Geometry check sheet. Reference: drawing and pictorial views, mm from the part's lowest x, y, z. A direction names the side the tool comes from. Coordinates: 2 decimals unless noted, no trailing zeros. Loops run counter-clockwise (first coordinate to the right, second up) from the corner with the lowest first, then second, coordinate; pieces in that order, holes last. Notation, with made-up numbers: M -36.5,40 L -22.5,40 A31 ccw -22.5,70 Z; hole C 56.5,81 d5. An arc over 180 degrees is marked long. Write item = value, one per line. Start each with the question number.
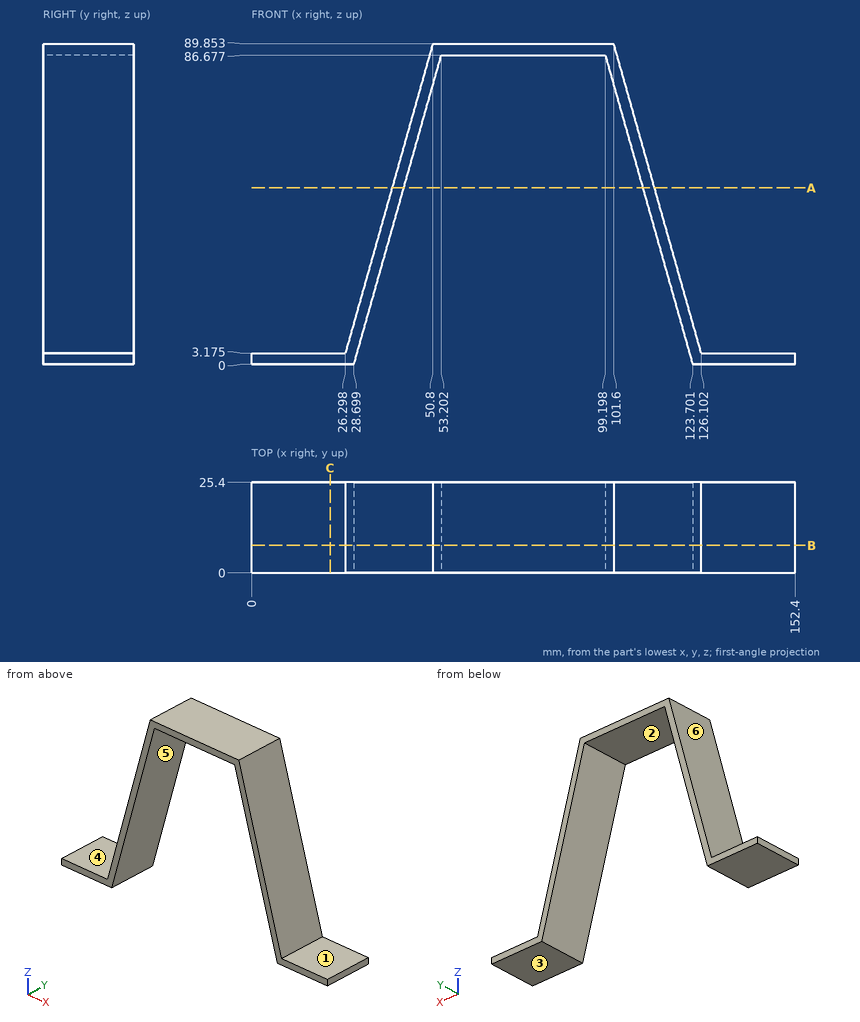
Q1. Scan lines: L1, parallel to Z at x = 13, y = 4.75 (1 decimal); L2, parallel to X at y = 8.5, z = 61 (1 decimal); L3, parallel to X at y = 1.75, z = 20 (1 decimal). Record each from-to range of solid material in increasing order. Write a range as [from, to].
Q2. Mould release check, pull along X, two halves, no side actions. Record for the marked faces 4, 5 and 6: +X half, -X half, draft (parallel to the pull), parting line (faces both ways), or undercut.
Q3. Sectioned sample at C-C on x = 22. Record the cut outline in (y, z) (1 decimal).
Q4. Gauge pin test, flat ends, axial feed: pin 1 (7.5 mm diameter, centred on x = 87.5, y = 16, fed in from -Z); pin 2 (1.5 mm diameter, centred on y = 17.5, z = 55.5, fed in from -X); pin 3 (12 mm diameter, centred on y = 9, z = 41, fed in from -X); pin 4 (12 mm diameter, centred on x = 96, z = 75, fed in from -Y). Record the tip position at first contact, or that the pin passes through.
Q5. Sectioned sample at B-B on y = 7.75. Record the cut outline in (x, z) (1 decimal).
Q6. Set-up check for the marked faces 1, 2 and 3: record each of +Z, -Z, +X, -X, +Y, -Y from which the full face is reachable in a straight line by a thin tool's end or side.
Q7. Sectioned sample at A-A on z = 49.5. Record the cut outline in (x, y).
Solutions:
q1.L1 = [0, 3.2]
q1.L2 = [42.6, 45.9], [106.5, 109.8]
q1.L3 = [31.1, 34.4], [118, 121.3]
q2.face_4 = draft
q2.face_5 = undercut
q2.face_6 = -X half
q3.outline = M 0,0 L 25.4,0 L 25.4,3.2 L 0,3.2 Z
q4.pin_1 = 86.68
q4.pin_2 = 40.88
q4.pin_3 = 35.29
q4.pin_4 = through
q5.outline = M 0,0 L 28.7,0 L 53.2,86.7 L 99.2,86.7 L 123.7,0 L 152.4,0 L 152.4,3.2 L 126.1,3.2 L 101.6,89.9 L 50.8,89.9 L 26.3,3.2 L 0,3.2 Z
q6.face_1 = +Z, +X, +Y, -Y
q6.face_2 = -Z, +Y, -Y
q6.face_3 = -Z, +X, -X, +Y, -Y
q7.outline = M 39.39,0 L 42.69,0 L 42.69,25.4 L 39.39,25.4 Z; M 109.71,0 L 113.01,0 L 113.01,25.4 L 109.71,25.4 Z
